Design review of the part built by this model. Coordinates are the model's own, in mm. Give positions to 0.01 mm unless a question says otherwise; leave off trailing zeros. Order: outer loops, then holes, each group sorted by start corner. A loop starts at its lowest first (then second) coordinate and runs counter-clockwise, first axis right, second up. Notation, with made-up numbers: M 27,83.5 L 40,83.5 A10 cw 40,98.5 Z; hole C 3,41.25 d5. An arc over 180 degrees is marked long. Answer as a JSON object with one key per item and string values.
from build123d import *

# Parameters (mm, degrees)
SKETCH_1_R               = 30
SKETCH_1_R_2             = 3
EXTRUDE_1_DEPTH          = 10
CUT_EXTRUDE_1_DEPTH      = 44.588989435
CUT_EXTRUDE_1_DEPTH_BACK = 44.588989435
SKETCH_2_R               = 4
SKETCH_3_R               = 2
EXTRUDE_2_DEPTH          = 32.5
HOLE_WIZARD_M5_2_D       = 4.2


with BuildPart() as part:
    # 草图1 → 凸台-拉伸1 (new body)
    with BuildSketch(Plane(origin=(0, 0, 0), x_dir=(1, 0, 0), z_dir=(0, 1, 0))):
        with Locations(Location((0, 0, 0), (0, 0, 270))):
            Circle(SKETCH_1_R)
        with Locations(Location((-17.67766953, 17.67766953, 0), (0, 0, 270))):
            Circle(SKETCH_1_R_2, mode=Mode.SUBTRACT)
        with Locations(Location((17.67766953, 17.67766953, 0), (0, 0, 90))):
            Circle(SKETCH_1_R_2, mode=Mode.SUBTRACT)
        with Locations(Location((17.67766953, -17.67766953, 0), (0, 0, 270))):
            Circle(SKETCH_1_R_2, mode=Mode.SUBTRACT)
        with Locations(Location((-17.67766953, -17.67766953, 0), (0, 0, 90))):
            Circle(SKETCH_1_R_2, mode=Mode.SUBTRACT)
    extrude(amount=EXTRUDE_1_DEPTH)

    # 草图2 → 切除-拉伸1 (cut, two sides: drawn at the far end of the back side and taken through both)
    with BuildSketch(Plane.XY.offset(-CUT_EXTRUDE_1_DEPTH_BACK)):
        with Locations((0, 5)):
            Circle(SKETCH_2_R)
    extrude(amount=CUT_EXTRUDE_1_DEPTH + CUT_EXTRUDE_1_DEPTH_BACK, mode=Mode.SUBTRACT)

    # 草图3 → 凸台-拉伸2 (add, symmetric)
    with BuildSketch(Plane(origin=(0, 0, 0), x_dir=(0, 0, -1), z_dir=(1, 0, 0))):
        with Locations(Location((0, 5, 0), (0, 0, 180))):
            Circle(SKETCH_3_R)
    extrude(amount=EXTRUDE_2_DEPTH, both=True)

    # M5 螺纹孔2 (through all)
    with Locations(Plane(origin=(32.5, 0, 0), x_dir=(0, 0, -1), z_dir=(1, 0, 0))):
        with Locations((0, 5)):
            Hole(HOLE_WIZARD_M5_2_D / 2)


solid = part.part
(1) We need section C-C (y = 3.75). Write out the cut boundary in (x, z).
Checked values:
{"outline": "M -29.95,-1.69 A30 ccw -3.8,-29.76 L -3.8,-1.69 Z; M -29.95,1.69 L -3.8,1.69 L -3.8,29.76 A30 ccw Z; M 3.8,-29.76 A30 ccw 29.95,-1.69 L 3.8,-1.69 Z; M 3.8,1.69 L 29.95,1.69 A30 ccw 3.8,29.76 Z; hole C -17.68,-17.68 d6; hole C -17.68,17.68 d6; hole C 17.68,-17.68 d6; hole C 17.68,17.68 d6"}
(2) Insertion check: pin 1 (2.5 mm diameter, centred on y = 5, z = 0, fed in from -X); pin 2 (1.5 mm diameter, centred on y = 7.5, z = -16, fed in from -X). Each pin has a flat end and moves straight along its axis. Give the tip position at first contact, or say it passes through.
Checked values:
{"pin 1": "passes through", "pin 2": "stops at x = -25.83"}
(3) To check wall thickness, follow L1, parallel to Y at x = 0, z = 3; L2, parallel to X at y = 2.75, z = -15; L3, parallel to X at y = 3, z = 17.5. State the ranges of each line that lie inside material, in increasing order. Write a range as from..to.
Checked values:
{"L1": "y = 0..1, 9..10", "L2": "x = -25.98..-19.03, -16.32..-3.31, 3.31..16.32, 19.03..25.98", "L3": "x = -24.37..-20.67, -14.68..-3.46, 3.46..14.68, 20.67..24.37"}
(4) We need section B-B (x = 16). Write out the cut boundary in (y, z).
Checked values:
{"outline": "M 0,-25.38 L 10,-25.38 L 10,-20.16 L 0,-20.16 Z; M 0,-15.19 L 10,-15.19 L 10,15.19 L 0,15.19 Z; M 0,20.16 L 10,20.16 L 10,25.38 L 0,25.38 Z; hole C 5,0 d4.2"}
(5) Draft analysis for pull direction X (two halves, no side actions). For faces 1 (the cylindrical face through (-11.49, 4.93, 27.712)), 2 (the flat face through (0, 10, 0)), 3 (the cylindrical face through (-19.5, 4.93, -20.06)), state which applies: +X half, -X half, draft (parallel to the pull), parting line (faces both ways), or undercut.
Checked values:
{"face 1": "parting line", "face 2": "draft", "face 3": "undercut"}
(6) We need section A-A (z = 0). Write out the cut boundary in (x, y), plus the area to 3 significant figures.
Checked values:
{"outline": "M -30,0 L 30,0 L 30,2.9 L 3.4,2.9 A4 cw -3.4,2.9 L -30,2.9 Z; M -30,7.1 L -3.4,7.1 A4 cw 3.4,7.1 L 30,7.1 L 30,10 L -30,10 Z", "area": "330 mm^2"}
(7) We need section D-D (z = 19). Write out the cut boundary in (x, y).
Checked values:
{"outline": "M -23.22,0 L -20.37,0 L -20.37,10 L -23.22,10 Z; M -14.98,0 L 14.98,0 L 14.98,10 L -14.98,10 Z; M 20.37,0 L 23.22,0 L 23.22,10 L 20.37,10 Z; hole C 0,5 d8"}
